Verification items for this drawing (mm, ordinates from the low corner). A direction names the side the tool comes from. Give positions to 0.01 mm unless a question says otherwise; leave off trailing zeros. Order: outer loops, then holes, each group sorted by start corner. A loop starts at its lowest first (then second) coordinate and runs counter-clockwise, first axis right, second up.
(1) Sectioned sample at A-A on y = 11. Record the cut outline in (x, z).
(2) Sectioned sample at B-B on x = 283. Record the cut outline in (y, z), plus the area to 3 significant figures.
(3) Sectioned sample at C-C on z = 59. Record the cut outline in (x, y), plus the area to 3 significant figures.
(4) Access from +Z, -Z, +X, -X, +Y, -Y to the whole of each face (thin tool, end or side, straight path). Record for the marked faces 4, 5 and 6.
(5) Scan lines: L1, parallel to X at y = 15.5, z = 81; L2, parallel to Z at x = 52, y = 8.25; L3, parallel to Z at x = 188, y = 11.75. Record each from-to range of solid material in increasing order.
(6) Gauge pin test, flat ends, axial feed: pin 1 (4 mm diameter, centred on y = 6.5, z = 59.5, fed in from +X); pin 2 (3 mm diameter, centred on x = 249, z = 21, fed in from -Y); pin 3 (1.5 mm diameter, centred on y = 12.5, z = 50, fed in from -X); pin 4 (2.5 mm diameter, centred on x = 188, z = 81, fed in from +Y). Record the tip position at first contact, or that the pin passes through.
(7) Mould release check, pull along Z, two halves, no side actions. Record for the marked faces 1, 2 and 3: pulls with the +Z half, pulls with the -Z half, needs draft (parallel to the pull), parting line crosses it, or undercut.
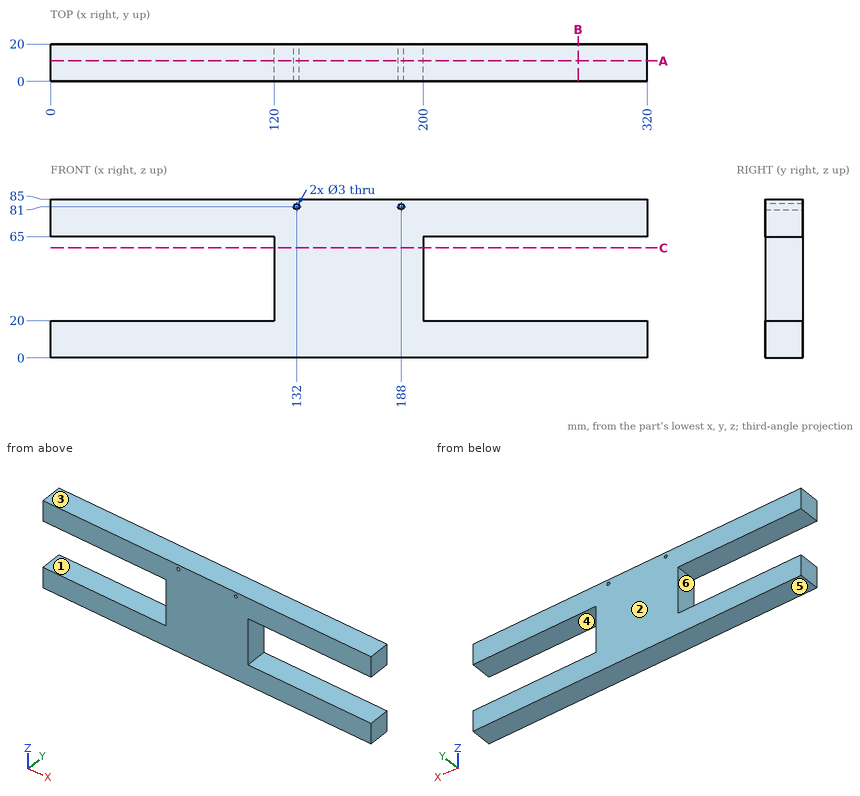
Ans:
1. outline: (0, 0) - (320, 0) - (320, 20) - (200, 20) - (200, 65) - (320, 65) - (320, 85) - (0, 85) - (0, 65) - (120, 65) - (120, 20) - (0, 20) - close; hole circle Ø3 at (132, 81); hole circle Ø3 at (188, 81)
2. outline: (0, 0) - (20, 0) - (20, 20) - (0, 20) - close; (0, 65) - (20, 65) - (20, 85) - (0, 85) - close
2. area: 800 mm2
3. outline: (120, 0) - (200, 0) - (200, 20) - (120, 20) - close
3. area: 1,600 mm2
4. face 4: +X, +Y, -Y
4. face 5: -Z, +X, -X, +Y, -Y
4. face 6: -X, +Y, -Y
5. L1: x = 0 to 130.5, 133.5 to 186.5, 189.5 to 320
5. L2: z = 0 to 20, 65 to 85
5. L3: z = 0 to 79.5, 82.5 to 85
6. pin 1: stops at x = 200
6. pin 2: stops at y = 0
6. pin 3: stops at x = 120
6. pin 4: passes through
7. face 1: undercut
7. face 2: needs draft
7. face 3: pulls with the +Z half
